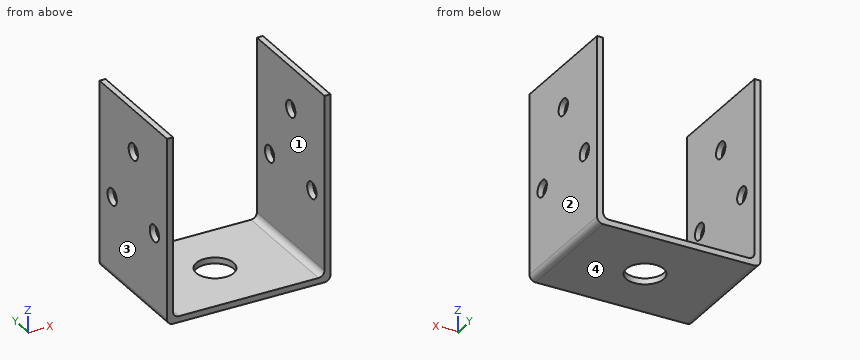
```python
from build123d import *

# Parameters (mm, degrees)
F1_DEPTH = 80
F2_R     = 12.5
F3_DEPTH = 4.001
F4_R     = 5.5
F5_DEPTH = 109.001
F6_R     = 4


with BuildPart() as f1:
    # F0 (on Front) → F1 (new body)
    with BuildSketch(Plane.XZ):
        Polygon((0, 0), (0, 120), (-4, 120), (-4, -4), (105, -4), (105, 120), (101, 120), (101, 0), align=None)
    extrude(amount=F1_DEPTH)

    # F2 (on face) → F3 (cut, through all)
    with BuildSketch(Plane.XY):
        with Locations((50.5, -40)):
            Circle(F2_R)
    extrude(amount=-F3_DEPTH, mode=Mode.SUBTRACT)

    # F4 (on face) → F5 (cut, through all)
    with BuildSketch(Plane(origin=(-4, 0, 0), x_dir=(0, -1, 0), z_dir=(-1, 0, 0))):
        with Locations((65, 50)):
            Circle(F4_R)
        with Locations((40, 92)):
            Circle(F4_R)
        with Locations((15, 50)):
            Circle(F4_R)
    extrude(amount=-F5_DEPTH, mode=Mode.SUBTRACT)

    # F6
    f6_edges = [f1.edges().sort_by_distance(p)[0] for p in [
        (0, -40, 0),
        (101, -40, 0),
        (-4, -40, -4),
        (105, -40, -4),
    ]]
    fillet(f6_edges, radius=F6_R)


solid = f1.part
```
Check sheet for the modelled part. Datum: model origin and axes. Units: mm. Face numbers are marked on the shaded views. Coordinates: 2 decimals unless noted, no trailing zeros. Order: outer loops, then holes, each group sorted by start corner. A loop starts at its lowest first (then second) coordinate and runs counter-clockwise, first axis right, second up. Notation, with made-up numbers: (85, -29) -> (140, -29) arc R15 cw to (140, -15) -> close; hole circle Ø4 at (-39, 5.5). An arc over 180 degrees is marked (long way). Write item = value, one per line. Start each with the question number.
1) Cross-section at B-B (y = -40). Enter the section's corners in (x, z).
2) Cross-section at A-A (z = 12). Enter the section's corners in (x, y), then the cut area to 3 significant figures.
3) Material ranges on L1, parallel to X at y = -67, z = 72.5; L2, parallel to Z at x = 29, y = -63.5; L3, parallel to Z at x = -2, y = -65, recorded low to high.
4) Go/stop test with a flat-tipped pin: P1, Ø1, axis at x = 73, y = -72, coming from the +Z side. Record where the tip stops, or that it passes through.
5) Cross-section at C-C (x = 50.5). Enter the section's corners in (y, z), then the cut area to 3 significant figures.
6) Cross-section at D-D (y = -15). Enter the section's corners in (x, z), then the cut area to 3 significant figures.
7) Mould release check, pull along X, two halves, no side actions. Record for the marked faces 1, 2, 3 and 4: +X half, -X half, draft (parallel to the pull), parting line (faces both ways), or undercut.
Ans:
q1.outline = (-4, 0) arc R4 ccw to (0, -4) -> (38, -4) -> (38, 0) -> (4, 0) arc R4 cw to (0, 4) -> (0, 86.5) -> (-4, 86.5) -> close; (-4, 97.5) -> (0, 97.5) -> (0, 120) -> (-4, 120) -> close; (63, -4) -> (101, -4) arc R4 ccw to (105, 0) -> (105, 86.5) -> (101, 86.5) -> (101, 4) arc R4 cw to (97, 0) -> (63, 0) -> close; (101, 97.5) -> (105, 97.5) -> (105, 120) -> (101, 120) -> close
q2.outline = (-4, -80) -> (0, -80) -> (0, 0) -> (-4, 0) -> close; (101, -80) -> (105, -80) -> (105, 0) -> (101, 0) -> close
q2.area = 640 mm²
q3.L1 = -4 to 0, 101 to 105
q3.L2 = -4 to 0
q3.L3 = -3.46 to 44.5, 55.5 to 120
q4.P1 = 0
q5.outline = (-80, -4) -> (-52.5, -4) -> (-52.5, 0) -> (-80, 0) -> close; (-27.5, -4) -> (0, -4) -> (0, 0) -> (-27.5, 0) -> close
q5.area = 220 mm²
q6.outline = (-4, 0) arc R4 ccw to (0, -4) -> (101, -4) arc R4 ccw to (105, 0) -> (105, 44.5) -> (101, 44.5) -> (101, 4) arc R4 cw to (97, 0) -> (4, 0) arc R4 cw to (0, 4) -> (0, 44.5) -> (-4, 44.5) -> close; (-4, 55.5) -> (0, 55.5) -> (0, 120) -> (-4, 120) -> close; (101, 55.5) -> (105, 55.5) -> (105, 120) -> (101, 120) -> close
q6.area = 1,310 mm²
q7.face_1 = undercut
q7.face_2 = +X half
q7.face_3 = -X half
q7.face_4 = draft
